from build123d import *

# Parameters (mm, degrees)
F0_DEPTH = 12.7
F1_R     = 2.5527
F2_DEPTH = 50.801
F3_SIZE  = 0.79375
F5_DEPTH = 12.701
F6_DEPTH = 12.7
F7_W     = 25.4
F7_H     = 12.7
F8_DEPTH = 25.4
F9_DEPTH = 12.7


# Not quite as in the source:
# - a feature names something its author has since deleted; it is built from what else it names


with BuildPart() as f0:
    # F10 (on Top) → F0 (new body)
    with BuildSketch(Plane.XY):
        Polygon((-71.4375, -15.875), (-71.4375, -25.4), (71.4375, -25.4), (71.4375, 25.4), (60.6425, 25.4), (60.6425, -12.7), (55.5625, -12.7), (55.5625, 25.4), (42.8625, 25.4), (42.8625, -12.7), (37.7825, -12.7), (37.7825, 25.4), (25.0825, 25.4), (25.0825, -12.7), (20.0025, -12.7), (20.0025, 25.4), (7.3025, 25.4), (7.3025, -12.7), (2.2225, -12.7), (2.2225, 25.4), (-10.4775, 25.4), (-10.4775, -12.7), (-15.5575, -12.7), (-15.5575, 25.4), (-28.2575, 25.4), (-28.2575, -12.7), (-33.3375, -12.7), (-33.3375, 25.4), (-71.4375, 25.4), (-71.4375, 15.875), (-46.0375, 15.875), (-46.0375, -15.875), align=None)
    extrude(amount=F0_DEPTH)

    # F1 (on face) → F2 (cut, through all)
    with BuildSketch(Plane.XZ.offset(25.4)):
        with Locations((-65.0875, 6.35)):
            Circle(F1_R)
    extrude(amount=-F2_DEPTH, mode=Mode.SUBTRACT)

    # F3
    f3_edges = [f0.edges().sort_by_distance(p)[0] for p in [
        (-67.6402, 15.875, 6.35),
        (-62.5348, 20.6375, 6.35),
        (-67.6402, 25.4, 6.35),
        (-67.6402, -25.4, 6.35),
        (-62.5348, -20.6375, 6.35),
        (-67.6402, -15.875, 6.35),
    ]]
    chamfer(f3_edges, length=F3_SIZE)

    # F4 (on face) → F5 (cut, through all)
    with BuildSketch(Plane.XY.offset(12.7)):
        with BuildLine():
            ThreePointArc((-46.0375, 14.2875), (-44.9149679849, 14.7524679849), (-44.45, 15.875))
            ThreePointArc((-44.45, 15.875), (-46.0375, 17.4625), (-47.625, 15.875))
            Line((-47.625, 15.875), (-46.0375, 15.875))
            Line((-46.0375, 15.875), (-46.0375, 14.2875))
        make_face()
        with BuildLine():
            ThreePointArc((-44.45, -15.875), (-44.9149679849, -14.7524679849), (-46.0375, -14.2875))
            Line((-46.0375, -14.2875), (-46.0375, -15.875))
            Line((-46.0375, -15.875), (-47.625, -15.875))
            ThreePointArc((-47.625, -15.875), (-46.0375, -17.4625), (-44.45, -15.875))
        make_face()
    extrude(amount=-F5_DEPTH, mode=Mode.SUBTRACT)

    # F4 (on face) → F6 (cut, through all)
    with BuildSketch(Plane.XY.offset(12.7)):
        with BuildLine():
            Line((-33.3375, -12.7), (-33.3375, -11.509375))
            ThreePointArc((-33.3375, -11.509375), (-34.1793990114, -13.5418990114), (-32.146875, -12.7))
            Line((-32.146875, -12.7), (-33.3375, -12.7))
        make_face()
        with BuildLine():
            Line((-28.2575, -12.7), (-29.448125, -12.7))
            ThreePointArc((-29.448125, -12.7), (-28.2575, -13.890625), (-27.066875, -12.7))
            ThreePointArc((-27.066875, -12.7), (-27.4156009886, -11.8581009886), (-28.2575, -11.509375))
            Line((-28.2575, -11.509375), (-28.2575, -12.7))
        make_face()
        with BuildLine():
            Line((-15.5575, -12.7), (-15.5575, -11.509375))
            ThreePointArc((-15.5575, -11.509375), (-16.3993990114, -13.5418990114), (-14.366875, -12.7))
            Line((-14.366875, -12.7), (-15.5575, -12.7))
        make_face()
        with BuildLine():
            Line((-10.4775, -12.7), (-11.668125, -12.7))
            ThreePointArc((-11.668125, -12.7), (-10.4775, -13.890625), (-9.286875, -12.7))
            ThreePointArc((-9.286875, -12.7), (-9.6356009886, -11.8581009886), (-10.4775, -11.509375))
            Line((-10.4775, -11.509375), (-10.4775, -12.7))
        make_face()
        with BuildLine():
            Line((2.2225, -12.7), (2.2225, -11.509375))
            ThreePointArc((2.2225, -11.509375), (1.3806009886, -13.5418990114), (3.413125, -12.7))
            Line((3.413125, -12.7), (2.2225, -12.7))
        make_face()
        with BuildLine():
            Line((7.3025, -12.7), (6.111875, -12.7))
            ThreePointArc((6.111875, -12.7), (7.3025, -13.890625), (8.493125, -12.7))
            ThreePointArc((8.493125, -12.7), (8.1443990114, -11.8581009886), (7.3025, -11.509375))
            Line((7.3025, -11.509375), (7.3025, -12.7))
        make_face()
        with BuildLine():
            Line((20.0025, -12.7), (20.0025, -11.509375))
            ThreePointArc((20.0025, -11.509375), (19.1606009886, -13.5418990114), (21.193125, -12.7))
            Line((21.193125, -12.7), (20.0025, -12.7))
        make_face()
        with BuildLine():
            ThreePointArc((26.273125, -12.7), (25.9243990114, -11.8581009886), (25.0825, -11.509375))
            Line((25.0825, -11.509375), (25.0825, -12.7))
            Line((25.0825, -12.7), (23.891875, -12.7))
            ThreePointArc((23.891875, -12.7), (25.0825, -13.890625), (26.273125, -12.7))
        make_face()
        with BuildLine():
            ThreePointArc((37.7825, -11.509375), (36.9406009886, -13.5418990114), (38.973125, -12.7))
            Line((38.973125, -12.7), (37.7825, -12.7))
            Line((37.7825, -12.7), (37.7825, -11.509375))
        make_face()
        with BuildLine():
            ThreePointArc((44.053125, -12.7), (43.7043990114, -11.8581009886), (42.8625, -11.509375))
            Line((42.8625, -11.509375), (42.8625, -12.7))
            Line((42.8625, -12.7), (41.671875, -12.7))
            ThreePointArc((41.671875, -12.7), (42.8625, -13.890625), (44.053125, -12.7))
        make_face()
        with BuildLine():
            ThreePointArc((55.5625, -11.509375), (54.7206009886, -13.5418990114), (56.753125, -12.7))
            Line((56.753125, -12.7), (55.5625, -12.7))
            Line((55.5625, -12.7), (55.5625, -11.509375))
        make_face()
        with BuildLine():
            ThreePointArc((61.833125, -12.7), (61.4843990114, -11.8581009886), (60.6425, -11.509375))
            Line((60.6425, -11.509375), (60.6425, -12.7))
            Line((60.6425, -12.7), (59.451875, -12.7))
            ThreePointArc((59.451875, -12.7), (60.6425, -13.890625), (61.833125, -12.7))
        make_face()
    extrude(amount=-F6_DEPTH, mode=Mode.SUBTRACT)

    # F7 (on face) → F8 (join)
    with BuildSketch(Plane.YZ.offset(71.4375)):
        with Locations((12.7, 6.35)):
            Rectangle(F7_W, F7_H)
    extrude(amount=F8_DEPTH)

    # F11 (on face) → F9 (cut, through all)
    with BuildSketch(Plane.XY.offset(12.7)):
        with BuildLine():
            Line((71.4375, 10.715625), (71.4375, 9.525))
            Line((71.4375, 9.525), (72.628125, 9.525))
            ThreePointArc((72.628125, 9.525), (72.2793990114, 10.3668990114), (71.4375, 10.715625))
        make_face()
        with BuildLine():
            Line((72.628125, 9.525), (71.4375, 9.525))
            Line((71.4375, 9.525), (71.4375, 10.715625))
            ThreePointArc((71.4375, 10.715625), (70.5956009886, 8.6831009886), (72.628125, 9.525))
        make_face()
        with BuildLine():
            ThreePointArc((71.4375, 10.715625), (72.2793990114, 10.3668990114), (72.628125, 9.525))
            Line((72.628125, 9.525), (96.8375, 9.525))
            Line((96.8375, 9.525), (96.8375, 13.335))
            Line((96.8375, 13.335), (93.3474382109, 13.335))
            ThreePointArc((93.3474382109, 13.335), (84.7328125, 11.1025068978), (76.1181867891, 13.335))
            Line((76.1181867891, 13.335), (71.4375, 13.335))
            Line((71.4375, 13.335), (71.4375, 10.715625))
        make_face()
        with BuildLine():
            Line((71.4375, 14.684375), (71.4375, 13.335))
            Line((71.4375, 13.335), (76.1181867891, 13.335))
            ThreePointArc((76.1181867891, 13.335), (74.2956009479, 14.4984363954), (72.628125, 15.875))
            ThreePointArc((72.628125, 15.875), (72.2793990114, 15.0331009886), (71.4375, 14.684375))
        make_face()
        with BuildLine():
            Line((93.3474382109, 13.335), (96.8375, 13.335))
            Line((96.8375, 13.335), (96.8375, 15.875))
            ThreePointArc((96.8375, 15.875), (95.1700240521, 14.4984363954), (93.3474382109, 13.335))
        make_face()
        with BuildLine():
            ThreePointArc((71.4674857978, 17.0652473451), (70.2469694175, 15.8899940879), (71.4375, 14.684375))
            Line((71.4375, 14.684375), (71.4375, 15.875))
            Line((71.4375, 15.875), (72.628125, 15.875))
            ThreePointArc((72.628125, 15.875), (72.0338528048, 16.4565181579), (71.4674857978, 17.0652473451))
        make_face()
        with BuildLine():
            Line((71.4375, 15.875), (71.4375, 14.684375))
            ThreePointArc((71.4375, 14.684375), (72.2793990114, 15.0331009886), (72.628125, 15.875))
            Line((72.628125, 15.875), (71.4375, 15.875))
        make_face()
        with BuildLine():
            Line((71.4375, 0), (72.628125, 0))
            ThreePointArc((72.628125, 0), (70.5956009886, 0.8418990114), (71.4375, -1.190625))
            Line((71.4375, -1.190625), (71.4375, 0))
        make_face()
        with BuildLine():
            ThreePointArc((75.0951666073, 15.875), (77.5332428869, 14.378226663), (80.1971168511, 13.335))
            Line((80.1971168511, 13.335), (89.2685081489, 13.335))
            ThreePointArc((89.2685081489, 13.335), (91.9323821131, 14.378226663), (94.3704583927, 15.875))
            Line((94.3704583927, 15.875), (75.0951666073, 15.875))
        make_face()
        with BuildLine():
            Line((89.2685081489, 13.335), (80.1971168511, 13.335))
            ThreePointArc((80.1971168511, 13.335), (84.7328125, 12.6851833333), (89.2685081489, 13.335))
        make_face()
    extrude(amount=-F9_DEPTH, mode=Mode.SUBTRACT)


solid = f0.part
Here's how the part is built. I have some questions about the finished solid (model axes, mm). A direction names the side the tool comes from. Round coordinates to 2 decimals unless told otherwise and drop trailing zeros. Loops run counter-clockwise (first coordinate to the right, second up) from the corner with the lowest first, then second, coordinate; pieces in that order, holes last. Notation, with made-up numbers: (32.5, 27.25) - (78.5, 27.25) arc R21 ccw to (78.5, 31.25) - close; hole circle Ø7 at (-26, 77). An arc over 180 degrees is marked (long way). One line per question, with ' | ' between items. Start each with the question number.
Q1. I want a section at A-A (y = -6). Write out the boundary of the cut face in (x, z), then the cut area to 3 significant figures.
Q2. Will these pins go through, and if not, where does the flat tip stop? pin 1 (4 mm diameter, centred on y = -7.5, z = 4, fed in from +X); pin 2 (0.8 mm diameter, centred on x = 4.5, z = 9, fed in from +Y); pin 3 (1.2 mm diameter, centred on y = 13.5, z = 6.5, fed in from +X).
Q3. Please list where these lines run through material, in increasing order: line 1 (Y direction, x = -28, z = 6); line 2 (Y direction, x = -63, z = 8.5); line 3 (Y direction, x = 5.5, z = 4). Write a range as [from, to].
Q4. I want a section at B-B (z = 6.35). State how many separate pieces and enclosed holes the cut face has, then the cut area to 3 significant figures.
Q5. For faces 1 (the flat face through (-60, 15.875, 6)), 2 (the flat face through (85, 15.875, 6)), 3 (the flat face through (85, 0, 6)), 4 (the flat face through (60.642, 7, 6)), which set-ups out of +Z, -Z, +X, -X, +Y, -Y let a thin tool reach every point of the face, with its end or its side?
Response values:
1) outline: (-46.04, 0) - (-33.34, 0) - (-33.34, 12.7) - (-46.04, 12.7) - close; (-28.26, 0) - (-15.56, 0) - (-15.56, 12.7) - (-28.26, 12.7) - close; (-10.48, 0) - (2.22, 0) - (2.22, 12.7) - (-10.48, 12.7) - close; (7.3, 0) - (20, 0) - (20, 12.7) - (7.3, 12.7) - close; (25.08, 0) - (37.78, 0) - (37.78, 12.7) - (25.08, 12.7) - close; (42.86, 0) - (55.56, 0) - (55.56, 12.7) - (42.86, 12.7) - close; (60.64, 0) - (71.44, 0) - (71.44, 12.7) - (60.64, 12.7) - close | area: 1,100 mm²
2) pin 1: stops at x = 71.44 | pin 2: stops at y = -12.7 | pin 3: stops at x = 94.6
3) line 1: y = [-25.4, -13.86], [-11.54, 25.4] | line 2: y = [-25.05, -16.22], [16.22, 25.05] | line 3: y = [-25.4, -12.7]
4) separate pieces: 3 | enclosed holes: 1 | area: 5,650 mm²
5) face 1: +Z, -Z, -X | face 2: +Z, -Z | face 3: +Z, -Z, +X, -Y | face 4: +Z, -Z, +Y
